```python
from build123d import *

# Parameters (mm, degrees)
F0_R     = 5
F1_DEPTH = 33
F2_R     = 6
F3_DEPTH = 2
F4_R     = 3.75
F5_DEPTH = 35.001


with BuildPart() as f1:
    # F0 (on Top) → F1 (new body)
    with BuildSketch(Plane.XY):
        Circle(F0_R)
    extrude(amount=F1_DEPTH)

    # F2 (on face) → F3 (join)
    with BuildSketch(Plane(origin=(0, 0, 0), x_dir=(1, 0, 0), z_dir=(0, 0, -1))):
        Circle(F2_R)
    extrude(amount=F3_DEPTH)

    # F4 (on face) → F5 (cut, through all)
    with BuildSketch(Plane(origin=(0, 0, -2), x_dir=(1, 0, 0), z_dir=(0, 0, -1))):
        Circle(F4_R)
    extrude(amount=-F5_DEPTH, mode=Mode.SUBTRACT)


solid = f1.part
```
Build history of the part. All positions in model axes, mm. Round coordinates to 2 decimals unless told otherwise and drop trailing zeros. Order: outer loops, then holes, each group sorted by start corner. A loop starts at its lowest first (then second) coordinate and runs counter-clockwise, first axis right, second up. Notation, with made-up numbers: (28.25, 81.25) -> (84.25, 81.25) arc R18 ccw to (84.25, 98.25) -> close; hole circle Ø9 at (-13, 84.25). An arc over 180 degrees is marked (long way). Answer in a Markdown table with one row per item.
1) Wall check: L1, parallel to Y at x = -0.25, z = 3.5; L2, parallel to X at y = -3, z = 28.5; L3, parallel to Z at x = 1.25, y = -5. Give the ranges that are in metal, low to high.
Values:
| item | result |
|---|---|
| L1 | -4.99 to -3.74, 3.74 to 4.99 |
| L2 | -4 to -2.25, 2.25 to 4 |
| L3 | -2 to 0 |
2) Band-saw the part on D-D on z = 29. Give the cut face in (x, y), and give its area (3 significant figures).
Values:
| item | result |
|---|---|
| outline | circle Ø10 at (0, 0); hole circle Ø7.5 at (0, 0) |
| area | 34.4 mm2 |
3) Pin check, flat tips, straight feed: P1, Ø5, axis at x = -4, z = 28, coming from the -Y side; P2, Ø1.5, axis at x = 3, z = 13.5, coming from the -Y side; P3, Ø6, axis at x = 4.5, z = 16, coming from the +Y side; P4, Ø2, axis at x = 0, y = 2.5, coming from the -Z side. Stop position of each tip, or through.
Values:
| item | result |
|---|---|
| P1 | y = -4.77 |
| P2 | y = -4.47 |
| P3 | y = 4.77 |
| P4 | through |
4) Band-saw the part on C-C on x = 4.25. Give the cut face in (y, z), and give its area (3 significant figures).
Values:
| item | result |
|---|---|
| outline | (-4.24, -2) -> (4.24, -2) -> (4.24, 0) -> (2.63, 0) -> (2.63, 33) -> (-2.63, 33) -> (-2.63, 0) -> (-4.24, 0) -> close |
| area | 191 mm2 |
5) Band-saw the part on A-A on y = 0. Give the cut face in (x, z).
Values:
| item | result |
|---|---|
| outline | (-6, -2) -> (-3.75, -2) -> (-3.75, 33) -> (-5, 33) -> (-5, 0) -> (-6, 0) -> close; (3.75, -2) -> (6, -2) -> (6, 0) -> (5, 0) -> (5, 33) -> (3.75, 33) -> close |
6) Mould opens along Y. For faces 1 (the cylindrical face through (-1.08, -4.88, 16.27)), 2 (the flat face through (-4, -4, 0)), 3 (the cylindrical face through (-3.746, -0.165, 15.255)) say: released by +Y, released by -Y, zero draft, split by the parting line, or undercut.
Values:
| item | result |
|---|---|
| face 1 | split by the parting line |
| face 2 | zero draft |
| face 3 | undercut |
